```python
from build123d import *

# Parameters (mm, degrees)
F0_W     = 80
F0_H     = 80
F1_DEPTH = 20
F3_DEPTH = 15
F5_DEPTH = 10
F6_R     = 4
F7_DEPTH = 20.001


with BuildPart() as f1:
    # F0 (on Front) → F1 (new body)
    with BuildSketch(Plane.XZ):
        with Locations((-5, -40)):
            Rectangle(F0_W, F0_H)
    extrude(amount=F1_DEPTH)

    # F2 (on face) → F3 (cut)
    with BuildSketch(Plane(origin=(0, 0, 0), x_dir=(-1, 0, 0), z_dir=(0, 1, 0))):
        with BuildLine():
            ThreePointArc((-26, -56), (-24.242641, -60.242641), (-20, -62))
            Line((-20, -62), (20, -62))
            ThreePointArc((20, -62), (24.242641, -60.242641), (26, -56))
            Line((26, -56), (26, -16))
            ThreePointArc((26, -16), (24.242641, -11.757359), (20, -10))
            Line((20, -10), (-20, -10))
            ThreePointArc((-20, -10), (-24.242641, -11.757359), (-26, -16))
            Line((-26, -16), (-26, -56))
        make_face()
    extrude(amount=-F3_DEPTH, mode=Mode.SUBTRACT)

    # F4 (on face) → F5 (cut)
    with BuildSketch(Plane(origin=(0, 0, 0), x_dir=(-1, 0, 0), z_dir=(0, 1, 0))):
        with BuildLine():
            ThreePointArc((-30, -56), (-27.071068, -63.071068), (-20, -66))
            Line((-20, -66), (20, -66))
            ThreePointArc((20, -66), (27.071068, -63.071068), (30, -56))
            Line((30, -56), (30, -16))
            ThreePointArc((30, -16), (27.071068, -8.928932), (20, -6))
            Line((20, -6), (-20, -6))
            ThreePointArc((-20, -6), (-27.071068, -8.928932), (-30, -16))
            Line((-30, -16), (-30, -56))
        make_face()
    extrude(amount=-F5_DEPTH, mode=Mode.SUBTRACT)

    # F6 (on face) → F7 (cut, through all)
    with BuildSketch(Plane(origin=(0, 0, 0), x_dir=(-1, 0, 0), z_dir=(0, 1, 0))):
        with Locations((-20, -72)):
            Circle(F6_R)
        with Locations((20, -72)):
            Circle(F6_R)
    extrude(amount=-F7_DEPTH, mode=Mode.SUBTRACT)


solid = f1.part
```
Source: CAD feature listing. Evaluate the final solid. Frame: model axes, mm. A direction names the side the tool comes from. Coordinates: 2 decimals unless noted, no trailing zeros. Order: outer loops, then holes, each group sorted by start corner. A loop starts at its lowest first (then second) coordinate and runs counter-clockwise, first axis right, second up. Notation, with made-up numbers: (31, 74.5) - (77, 74.5) arc R14 ccw to (77, 95.5) - close; hole circle Ø9 at (83, -27.75). An arc over 180 degrees is marked (long way). One line per item, written item: value.
1) Contact query for flat-ended pins moving along their axis: pin 1 (4 mm diameter, centred on x = -13, z = -31.5, fed in from +Y); pin 2 (3 mm diameter, centred on x = -2.5, y = -4.5, fed in from +Z). Output: stop coordinate, or through.
Computed values:
pin 1: stops at y = -15
pin 2: stops at z = 0
2) Cut plane B-B on z = -72. Output: boundary loops of the cut face in (x, y), plus the area to 3 significant figures.
Computed values:
outline: (-45, -20) - (-24, -20) - (-24, 0) - (-45, 0) - close; (-16, -20) - (16, -20) - (16, 0) - (-16, 0) - close; (24, -20) - (35, -20) - (35, 0) - (24, 0) - close
area: 1,280 mm^2
3) Cut plane C-C on x = 11.5. Output: boundary loops of the cut face in (y, z), plus the area to 3 significant figures.
Computed values:
outline: (-20, -80) - (0, -80) - (0, -66) - (-10, -66) - (-10, -62) - (-15, -62) - (-15, -10) - (-10, -10) - (-10, -6) - (0, -6) - (0, 0) - (-20, 0) - close
area: 740 mm^2
4) Mould query, pull axis X, two halves, no side actions, for faces 3 (the face through (-45, -10, -41)), 4 (the face through (-24.196, -12.465, -60.289)), 5 (the face through (-6, -20, -39)). Classes: released by +X, released by -X, zero draft, split by the parting line, or undercut.
Computed values:
face 3: released by -X
face 4: undercut
face 5: zero draft
5) Ray query, line 1 (Z direction, x = 20, y = -13.75); line 2 (Z direction, x = 20, y = -9.75); line 3 (Z direction, x = -4.5, y = -5.25). Return the intervals inside material, ascending. Write a range as [from, to].
Computed values:
line 1: z = [-80, -76], [-68, -62], [-10, 0]
line 2: z = [-80, -76], [-68, -66], [-6, 0]
line 3: z = [-80, -66], [-6, 0]
6) Cut plane A-A on y = -14. Output: boundary loops of the cut face in (x, z), plus the area to 3 significant figures.
Computed values:
outline: (-45, -80) - (35, -80) - (35, 0) - (-45, 0) - close; hole (-26, -56) arc R6 ccw to (-20, -62) - (20, -62) arc R6 ccw to (26, -56) - (26, -16) arc R6 ccw to (20, -10) - (-20, -10) arc R6 ccw to (-26, -16) - close; hole circle Ø8 at (-20, -72); hole circle Ø8 at (20, -72)
area: 3,630 mm^2
7) Reachability of faces 1 (the face through (-6, -10, -80)), 2 (the face through (0, -12, -62)) from +Z, -Z, +X, -X, +Y, -Y: full face, straight path, thin tool, end or side. Return the list, or none.
Computed values:
face 1: -Z, +X, -X, +Y, -Y
face 2: +Y
8) Cut plane D-D on y = -7.25. Output: boundary loops of the cut face in (x, z), plus the area to 3 significant figures.
Computed values:
outline: (-45, -80) - (35, -80) - (35, 0) - (-45, 0) - close; hole (-30, -56) arc R10 ccw to (-20, -66) - (20, -66) arc R10 ccw to (30, -56) - (30, -16) arc R10 ccw to (20, -6) - (-20, -6) arc R10 ccw to (-30, -16) - close; hole circle Ø8 at (-20, -72); hole circle Ø8 at (20, -72)
area: 2,790 mm^2
